Input: dimensioned drawing with shaded views. Units: mm. Origin: part minimum x, y, z. A direction names the side the tool comes from. Round coordinates to 2 decimals unless told otherwise and drop trailing zeros. Loops run counter-clockwise (first coordinate to the right, second up) from the corner with the lowest first, then second, coordinate; pieces in that order, holes last. Notation, with made-up numbers: (31, 42.25) - (87, 42.25) arc R29 cw to (87, 79.25) - close; hole circle Ø4 at (87.5, -24.75). An arc over 180 degrees is marked (long way). Answer as CSV lines item,"result".
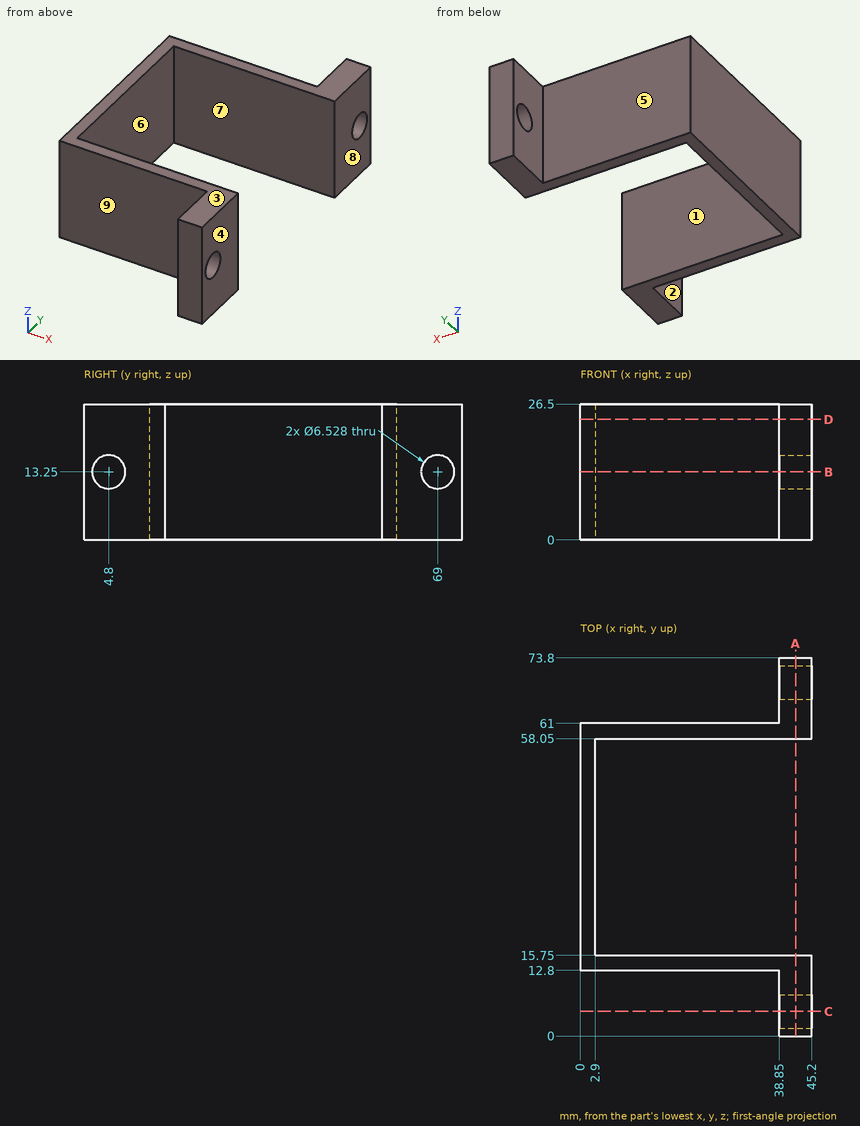
(1) Material intervals for line 1 along Y through (x, z) = (43.5, 13.5); line 2 along Z through (x, y) = (40, 69); line 3 along Y through (x, z) = (16, 25), sorted ascending.
Findings below:
line 1,"0 to 1.55, 8.05 to 15.75, 58.05 to 65.75, 72.25 to 73.8"
line 2,"0 to 9.99, 16.51 to 26.5"
line 3,"12.8 to 15.75, 58.05 to 61"
(2) Draft query along Y for the marked faces 6, 7, 8 and 9. Return one class per face: pulls with the +Y half, pulls with the -Y half, needs draft (parallel to the pull), parting line crosses it, or undercut.
Findings below:
face 6,"undercut"
face 7,"undercut"
face 8,"needs draft"
face 9,"pulls with the -Y half"
(3) Section B-B (z = 13.25). Output: boundary loops of the cut face in (x, y).
Findings below:
outline,"(0, 12.8) - (38.85, 12.8) - (38.85, 8.06) - (45.2, 8.06) - (45.2, 15.75) - (2.9, 15.75) - (2.9, 58.05) - (45.2, 58.05) - (45.2, 65.74) - (38.85, 65.74) - (38.85, 61) - (0, 61) - close; (38.85, 0) - (45.2, 0) - (45.2, 1.54) - (38.85, 1.54) - close; (38.85, 72.26) - (45.2, 72.26) - (45.2, 73.8) - (38.85, 73.8) - close"
(4) Section C-C (y = 4.8). Output: boundary loops of the cut face in (x, z).
Findings below:
outline,"(38.85, 0) - (45.2, 0) - (45.2, 9.99) - (38.85, 9.99) - close; (38.85, 16.51) - (45.2, 16.51) - (45.2, 26.5) - (38.85, 26.5) - close"
(5) Pin query (flat end, axial travel): P1, Ø4, axis at y = 4.8, z = 13.25, coming from the -X side; P2, Ø12, axis at x = 17, z = 9, coming from the +Y side; P3, Ø8, axis at x = 26.5, z = 14, coming from the -Y side; P4, Ø3, axis at y = 48, z = 16.5, coming from the +X side. Return the tip coordinate at first contact, or that it passes through.
Findings below:
P1,"through"
P2,"y = 61"
P3,"y = 12.8"
P4,"x = 2.9"
(6) Section A-A (x = 42). Output: boundary loops of the cut face in (y, z).
Findings below:
outline,"(0, 0) - (15.75, 0) - (15.75, 26.5) - (0, 26.5) - close; (58.05, 0) - (73.8, 0) - (73.8, 26.5) - (58.05, 26.5) - close; hole circle Ø6.53 at (4.8, 13.25); hole circle Ø6.53 at (69, 13.25)"
(7) Access query for the marked faces 1, 2, 3, 4 and 5. Directions: +Z, -Z, +X, -X, +Y, -Y. A direction counts if a zero-diameter tool reaches every point of the face in a straight line with its end or side. Return the directions, or none.
Findings below:
face 1,"+Z, -Z, +X"
face 2,"+Z, -Z, -X, -Y"
face 3,"+Z, +X, -X, +Y, -Y"
face 4,"+Z, -Z, +X, +Y, -Y"
face 5,"+Z, -Z, -X, +Y"
(8) Section D-D (z = 23.5). Output: boundary loops of the cut face in (x, y).
Findings below:
outline,"(0, 12.8) - (38.85, 12.8) - (38.85, 0) - (45.2, 0) - (45.2, 15.75) - (2.9, 15.75) - (2.9, 58.05) - (45.2, 58.05) - (45.2, 73.8) - (38.85, 73.8) - (38.85, 61) - (0, 61) - close"
